```python
from build123d import *

# Parameters (mm, degrees)
SKETCH1_R           = 4.7625
SKETCH1_R_2         = 4.03225
SKETCH1_R_3         = 1.524
SKETCH1_W           = 8.636
SKETCH1_H           = 4.7625
BOSS_EXTRUDE1_DEPTH = 4.7625


with BuildPart() as part:
    # Sketch1 → Boss-Extrude1 (new body)
    with BuildSketch(Plane(origin=(0, 0, 0), x_dir=(0, 0, -1), z_dir=(1, 0, 0))):
        with BuildLine():
            Line((42.1132, 8.7376), (42.1132, -18.894289209))
            Line((42.1132, -18.894289209), (28.215665755, -90.567816907))
            ThreePointArc((28.215665755, -90.567816907), (16.325222884, -100.837177304), (3.551201687, -91.690222777))
            Line((3.551201687, -91.690222777), (-17.5768, -18.894289209))
            Line((-17.5768, -18.894289209), (-17.5768, 8.7376))
            ThreePointArc((-17.5768, 8.7376), (-16.64686403, 10.98266403), (-14.4018, 11.9126))
            Line((-14.4018, 11.9126), (38.9382, 11.9126))
            ThreePointArc((38.9382, 11.9126), (41.18326403, 10.98266403), (42.1132, 8.7376))
        make_face()
        with Locations(Location((15.747881426, -88.15030705, 0), (0, 0, 180))):
            Circle(SKETCH1_R, mode=Mode.SUBTRACT)
        with Locations(Location((0, 0, 0), (0, 0, 180))):
            Circle(SKETCH1_R_2, mode=Mode.SUBTRACT)
        with Locations(Location((-12.78255, 4.3307, 0), (0, 0, 180))):
            Circle(SKETCH1_R_3, mode=Mode.SUBTRACT)
        with Locations(Location((36.2712, -3.8354, 0), (0, 0, 180))):
            Circle(SKETCH1_R_3, mode=Mode.SUBTRACT)
        with Locations(Location((-12.78255, -2.0193, 0), (0, 0, 180))):
            Circle(SKETCH1_R_3, mode=Mode.SUBTRACT)
        with Locations(Location((-12.78255, -8.3693, 0), (0, 0, 180))):
            Circle(SKETCH1_R_3, mode=Mode.SUBTRACT)
        with Locations(Location((19.5072, -3.8354, 0), (0, 0, 180))):
            Circle(SKETCH1_R_3, mode=Mode.SUBTRACT)
        with Locations((27.8892, -3.8354)):
            Rectangle(SKETCH1_W, SKETCH1_H, mode=Mode.SUBTRACT)
    extrude(amount=BOSS_EXTRUDE1_DEPTH)


solid = part.part
```
Here's how the part is built. I have some questions about the finished solid (model axes, mm). A direction names the side the tool comes from. Round coordinates to 2 decimals unless told otherwise and drop trailing zeros. Loops run counter-clockwise (first coordinate to the right, second up) from the corner with the lowest first, then second, coordinate; pieces in that order, holes last. Notation, with made-up numbers: (41, 11.25) -> (82, 11.25) arc R19 ccw to (82, 47.25) -> close; hole circle Ø9 at (67.25, 1). An arc over 180 degrees is marked (long way). Answer as CSV lines item,"result".
1. If we section it at C-C on x = 2.45: Count the separate pieces of the cut face and the enclosed holes in it, plus the area to 3 significant figures.
Final values:
separate pieces,"1"
enclosed holes,"8"
area,"4,860 mm^2"
2. For pin 1 (2.5 mm diameter, centred on y = -3.84, z = -19.51, fed in from +X); pin 2 (2.5 mm diameter, centred on x = 2, z = -25.5, fed in from -Y); pin 3 (2 mm diameter, centred on x = 2.5, y = -21.5, fed in from +Z), each with a flat end and sliding along its axis, tell me the tip position at first contact or that it passes through.
Final values:
pin 1,"passes through"
pin 2,"stops at y = -97.58"
pin 3,"stops at z = 17.11"
3. If we section it at B-B on y = 1.5: Please give me the cut outline in (x, z), plus the area to 3 significant figures.
Final values:
outline,"(0, -42.11) -> (4.76, -42.11) -> (4.76, -3.74) -> (0, -3.74) -> close; (0, 3.74) -> (4.76, 3.74) -> (4.76, 17.58) -> (0, 17.58) -> close"
area,"249 mm^2"
4. If I drill on L1, parallel to Y at x = 3.5, z = -24; L2, parallel to Z at x = 0.3, y = -35; L3, parallel to Z at x = 2.8, y = -89, over which ranges is the centre line in solid material (lowest first)?
Final values:
L1,"y = -97.8 to -6.22, -1.45 to 11.91"
L2,"z = -38.99 to 12.9"
L3,"z = -28.52 to -20.43, -11.06 to -2.77"
5. Thinking about a two-plate mould opening in Y: for faces 3 (the face through (2.348, -55.802, 6.865)), 4 (the face through (2.348, 11.007, -41.158)), 5 (the face through (2.35, -92.87, -16.37)), which applies, released by +Y, released by -Y, zero draft, split by the parting line, or undercut?
Final values:
face 3,"released by -Y"
face 4,"released by +Y"
face 5,"undercut"
6. If we section it at A-A on z = 0.5: Please give me the cut outline in (x, y), plus the area to 3 significant figures.
Final values:
outline,"(0, -77.73) -> (4.76, -77.73) -> (4.76, -4) -> (0, -4) -> close; (0, 4) -> (4.76, 4) -> (4.76, 11.91) -> (0, 11.91) -> close"
area,"389 mm^2"
7. Which directions (+Z, -Z, +X, -X, +Y, -Y) give clear straight access to the entire face, cutting with the end or side of a thin tool? Please do faces 1 (the face through (2, -4, -23.571)), 2 (the face through (4.762, -31, -13)).
Final values:
face 1,"+X, -X"
face 2,"+Z, -Z, +X, +Y, -Y"
8. If we section it at D-D on y = -77: Please give me the cut outline in (x, z).
Final values:
outline,"(0, -30.85) -> (4.76, -30.85) -> (4.76, 0.71) -> (0, 0.71) -> close"
